Can you work these out from the model? Positions are in its coordinate system, mm. Round coordinates to 2 decimals unless told otherwise and drop trailing zeros. Loops run counter-clockwise (first coordinate to the right, second up) from the corner with the lowest first, then second, coordinate; pieces in that order, holes last.
(1) I want a section at D-D on z = 70.5. Write out the boundary of the cut face in (x, y), plus the area to 3 significant figures.
(2) Thinking about a two-plate mould opening in Y: for faces 1 (the face through (0, -30, 37)), 2 (the face through (36.98, -21.057, 67.564)), 3 (the face through (37, 0, 37)), 4 (the face through (37, -74.82, 37)), which applies, released by +Y, released by -Y, zero draft, split by the parting line, or undercut?
(3) If I drill on line 1 along Z through (x, y) = (49, -13); line 2 along Z through (x, y) = (66.5, -9); line 3 along Y through (x, z) = (38.5, 70), over which ranges is the centre line in solid material (lowest first)?
(4) I want a section at C-C on x = 19.5. Give the number of separate pieces and of enclosed holes in the cut face, plus the area to 3 significant figures.
(5) I want a section at B-B on z = 10. Write out the boundary of the cut face in (x, y), plus the area to 3 significant figures.
(6) I want a section at A-A on y = -63. Write out the boundary of the cut face in (x, z), plus the area to 3 significant figures.
from build123d import *

# Parameters (mm, degrees)
F0_W     = 75.010031
F0_H     = 74.819528
F1_DEPTH = 74.9
F3_D     = 10


with BuildPart() as f1:
    # F0 (on Top) → F1 (new body)
    with BuildSketch(Plane.XY):
        with Locations((37.505015, -37.409764)):
            Rectangle(F0_W, F0_H)
    extrude(amount=F1_DEPTH)

    # F3 (through all)
    with Locations(Plane.YZ.offset(75.010031)):
        with Locations((-21.707887, 62.606953), (-40.798798, 38.462568), (-37.429813, 19.371659), (-66.627674, 67.09893), (-43.88703, 60.360968), (-12.723929, 27.51337), (-64.100936, 23.863638), (-10.197191, 7.580214)):
            Hole(F3_D / 2)


solid = f1.part
Filled sheet:
1. outline: (0, -74.82) - (75.01, -74.82) - (75.01, -70.29) - (0, -70.29) - close; (0, -62.96) - (75.01, -62.96) - (75.01, 0) - (0, 0) - close
1. area: 5,060 mm2
2. face 1: zero draft
2. face 2: undercut
2. face 3: released by +Y
2. face 4: released by -Y
3. line 1: z = 0 to 3.44, 11.72 to 22.52, 32.51 to 74.9
3. line 2: z = 0 to 2.73, 12.43 to 24.18, 30.85 to 74.9
3. line 3: y = -74.82 to -70.7, -62.56 to 0
4. separate pieces: 1
4. enclosed holes: 8
4. area: 4,980 mm2
5. outline: (0, -74.82) - (75.01, -74.82) - (75.01, -14.57) - (0, -14.57) - close; (0, -5.82) - (75.01, -5.82) - (75.01, 0) - (0, 0) - close
5. area: 4,960 mm2
6. outline: (0, 0) - (75.01, 0) - (75.01, 18.99) - (0, 18.99) - close; (0, 28.74) - (75.01, 28.74) - (75.01, 63.66) - (0, 63.66) - close; (0, 70.54) - (75.01, 70.54) - (75.01, 74.9) - (0, 74.9) - close
6. area: 4,370 mm2
